from build123d import *

# Parameters (mm, degrees)
ESBO_O1_W                = 500
ESBO_O1_H                = 460
ESBO_O1_R                = 10
RESSALTO_EXTRUS_O1_DEPTH = 4.7625


with BuildPart() as part:
    # Esboço1 → Ressalto-extrusão1 (new body)
    with BuildSketch(Plane.XY):
        with Locations((-100, 70)):
            Rectangle(ESBO_O1_W, ESBO_O1_H)
        with Locations(Location((0, 0, 0), (0, 0, 180))):
            Circle(ESBO_O1_R, mode=Mode.SUBTRACT)
        with Locations(Location((-100, 0, 0), (0, 0, 180))):
            Circle(ESBO_O1_R, mode=Mode.SUBTRACT)
        with Locations(Location((-200, 0, 0), (0, 0, 180))):
            Circle(ESBO_O1_R, mode=Mode.SUBTRACT)
        with Locations(Location((-200, 140, 0), (0, 0, 180))):
            Circle(ESBO_O1_R, mode=Mode.SUBTRACT)
        with Locations(Location((-100, 140, 0), (0, 0, 180))):
            Circle(ESBO_O1_R, mode=Mode.SUBTRACT)
        with Locations(Location((0, 140, 0), (0, 0, 180))):
            Circle(ESBO_O1_R, mode=Mode.SUBTRACT)
    extrude(amount=RESSALTO_EXTRUS_O1_DEPTH)


solid = part.part
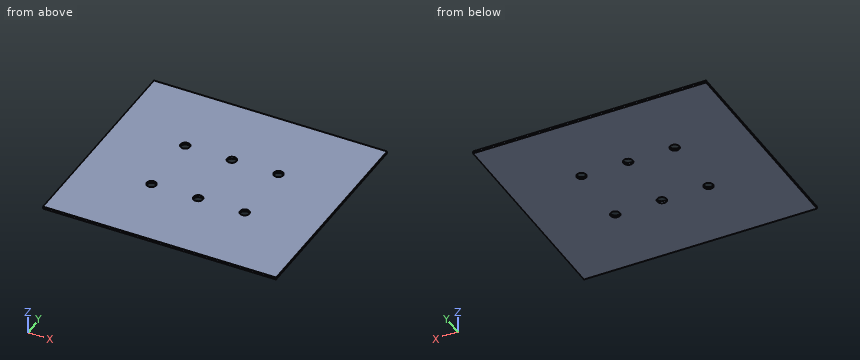
The model under review builds one solid part; all positions refer to its coordinate system, in mm. Give positions to 0.01 mm unless a question says otherwise; leave off trailing zeros. Loops run counter-clockwise (first coordinate to the right, second up) from the corner with the lowest first, then second, coordinate; pieces in that order, holes last. Notation, with made-up numbers: (44.5, 27) -> (84.5, 27) arc R26 ccw to (84.5, 66) -> close; hole circle Ø3 at (-25, 0.25). An arc over 180 degrees is marked (long way). Answer as a JSON object with one key per item and string values. Group by question number.
Q1. Take a section at A-A (x = 0). Write out the cut boundary in (y, z).
Q2. Wall thickness on line 1 along X through (y, z) = (140, 1.15); line 2 along Y through (x, z) = (0, 3.55); line 3 along X through (y, z) = (1, 0.7): over which ranges is each line inside the solid? List them lowest first.
Q3. Take a section at B-B (y = 140). Write out the cut boundary in (x, z), plus the area to 3 significant figures.
Answer below:
{
 "1": {"outline": "(-160, 0) -> (-10, 0) -> (-10, 4.76) -> (-160, 4.76) -> close; (10, 0) -> (130, 0) -> (130, 4.76) -> (10, 4.76) -> close; (150, 0) -> (300, 0) -> (300, 4.76) -> (150, 4.76) -> close"},
 "2": {"line 1": "x = -350 to -210, -190 to -110, -90 to -10, 10 to 150", "line 2": "y = -160 to -10, 10 to 130, 150 to 300", "line 3": "x = -350 to -209.95, -190.05 to -109.95, -90.05 to -9.95, 9.95 to 150"},
 "3": {"outline": "(-350, 0) -> (-210, 0) -> (-210, 4.76) -> (-350, 4.76) -> close; (-190, 0) -> (-110, 0) -> (-110, 4.76) -> (-190, 4.76) -> close; (-90, 0) -> (-10, 0) -> (-10, 4.76) -> (-90, 4.76) -> close; (10, 0) -> (150, 0) -> (150, 4.76) -> (10, 4.76) -> close", "area": "2,100 mm2"}
}
